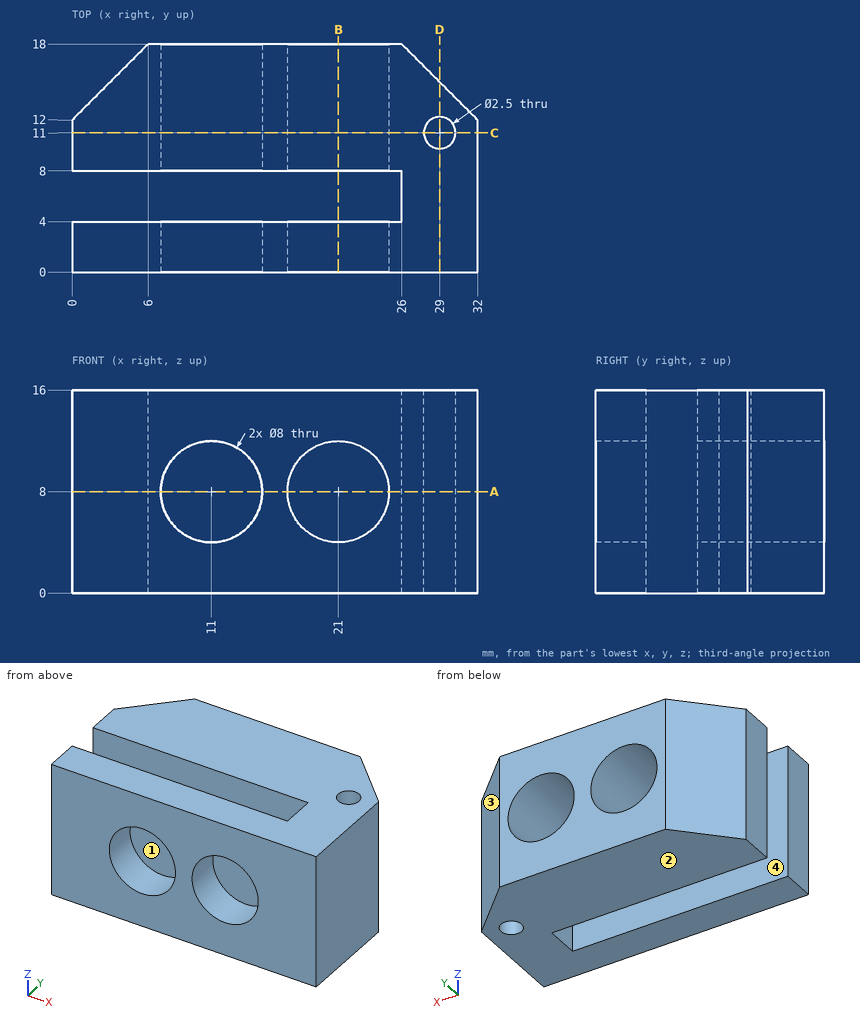
Geometry check sheet. Reference: drawing and pictorial views, mm from the part's lowest x, y, z. Coordinates: 2 decimals unless noted, no trailing zeros. Write each loop counter-clockwise with the first axis right and the second up, starting at its lowest first coordinate (ties: lowest second). Pieces come first, ordered by that corner, then holes. Notation, with made-up numbers: (21.25, 45) -> (30.25, 45) arc R26 ccw to (30.25, 66) -> close; hole circle Ø11 at (9.5, 25). An arc over 180 degrees is marked (long way). Use a Markdown table: item, result.
1. Sectioned sample at A-A (z = 8). Enter the section's corners in (x, y).
Reported:
| item | result |
|---|---|
| outline | (0, 0) -> (7, 0) -> (7, 4) -> (0, 4) -> close; (0, 8) -> (7, 8) -> (7, 18) -> (6, 18) -> (0, 12) -> close; (15, 0) -> (17, 0) -> (17, 4) -> (15, 4) -> close; (15, 8) -> (17, 8) -> (17, 18) -> (15, 18) -> close; (25, 0) -> (32, 0) -> (32, 12) -> (26, 18) -> (25, 18) -> (25, 8) -> (26, 8) -> (26, 4) -> (25, 4) -> close; hole circle Ø2.5 at (29, 11) |
2. Sectioned sample at D-D (x = 29). Enter the section's corners in (y, z).
Reported:
| item | result |
|---|---|
| outline | (0, 0) -> (9.75, 0) -> (9.75, 16) -> (0, 16) -> close; (12.25, 0) -> (15, 0) -> (15, 16) -> (12.25, 16) -> close |
3. Sectioned sample at B-B (x = 21). Enter the section's corners in (y, z), plus the area to 3 significant figures.
Reported:
| item | result |
|---|---|
| outline | (0, 0) -> (4, 0) -> (4, 4) -> (0, 4) -> close; (0, 12) -> (4, 12) -> (4, 16) -> (0, 16) -> close; (8, 0) -> (18, 0) -> (18, 4) -> (8, 4) -> close; (8, 12) -> (18, 12) -> (18, 16) -> (8, 16) -> close |
| area | 112 mm2 |
4. Go/stop test with a flat-tipped pin: pin 1 Ø5 at (x, z) = (11, 8) entering from +Y (1 decimal). Record where the tip stops, or that it passes through.
Reported:
| item | result |
|---|---|
| pin 1 | passes through |
5. Scan lines: line 1 along X through (y, z) = (1.3, 8); line 2 along Y through (x, z) = (5, 3.25); line 3 along Y through (x, z) = (14, 3). Record each from-to range of solid material in increasing order.
Reported:
| item | result |
|---|---|
| line 1 | x = 0 to 7, 15 to 17, 25 to 32 |
| line 2 | y = 0 to 4, 8 to 17 |
| line 3 | y = 0 to 4, 8 to 18 |
6. Release check for a two-part mould opening along Y. For the marked faces 1, 2, 3 and 4 record: pulls with the +Y half, pulls with the -Y half, needs draft (parallel to the pull), parting line crosses it, or undercut.
Reported:
| item | result |
|---|---|
| face 1 | undercut |
| face 2 | needs draft |
| face 3 | pulls with the +Y half |
| face 4 | undercut |
7. Sectioned sample at C-C (y = 11). Enter the section's corners in (x, z).
Reported:
| item | result |
|---|---|
| outline | (0, 0) -> (27.75, 0) -> (27.75, 16) -> (0, 16) -> close; (30.25, 0) -> (32, 0) -> (32, 16) -> (30.25, 16) -> close; hole circle Ø8 at (11, 8); hole circle Ø8 at (21, 8) |
